```python
from build123d import *

# Parameters (mm, degrees)
EXTRUDE_F_DEPTH    = 736.6
CUT_EXTRUDE1_REACH = 740.684
SKETCH2_R          = 2.667


with BuildPart() as part:
    # Sketch1 → Extrude f (new body)
    with BuildSketch(Plane.XY):
        Polygon((3.175, 3.175), (3.175, 25.4), (0, 25.4), (0, 0), (50.8, 0), (50.8, 25.4), (47.625, 25.4), (47.625, 3.175), align=None)
    extrude(amount=EXTRUDE_F_DEPTH)

    # Sketch2 → Cut-Extrude1 (cut, up to next)
    with BuildSketch(Plane(origin=(0, 3.175, 0), x_dir=(1, 0, 0), z_dir=(0, 1, 0)), mode=Mode.PRIVATE) as cut_extrude1_sk1:
        with Locations(Location((12.7, -723.9, 0), (0, 0, 270))):
            Circle(SKETCH2_R)
    cut_extrude1_tool1 = extrude(cut_extrude1_sk1.sketch, amount=-CUT_EXTRUDE1_REACH, mode=Mode.PRIVATE) & part.part
    # Sketch2 → Cut-Extrude1 (cut, up to next)
    with BuildSketch(Plane(origin=(0, 3.175, 0), x_dir=(1, 0, 0), z_dir=(0, 1, 0)), mode=Mode.PRIVATE) as cut_extrude1_sk2:
        with Locations(Location((12.7, -660.4, 0), (0, 0, 270))):
            Circle(SKETCH2_R)
    cut_extrude1_tool2 = extrude(cut_extrude1_sk2.sketch, amount=-CUT_EXTRUDE1_REACH, mode=Mode.PRIVATE) & part.part
    # Sketch2 → Cut-Extrude1 (cut, up to next)
    with BuildSketch(Plane(origin=(0, 3.175, 0), x_dir=(1, 0, 0), z_dir=(0, 1, 0)), mode=Mode.PRIVATE) as cut_extrude1_sk3:
        with Locations(Location((38.1, -660.4, 0), (0, 0, 270))):
            Circle(SKETCH2_R)
    cut_extrude1_tool3 = extrude(cut_extrude1_sk3.sketch, amount=-CUT_EXTRUDE1_REACH, mode=Mode.PRIVATE) & part.part
    # Sketch2 → Cut-Extrude1 (cut, up to next)
    with BuildSketch(Plane(origin=(0, 3.175, 0), x_dir=(1, 0, 0), z_dir=(0, 1, 0)), mode=Mode.PRIVATE) as cut_extrude1_sk4:
        with Locations(Location((38.1, -723.9, 0), (0, 0, 270))):
            Circle(SKETCH2_R)
    cut_extrude1_tool4 = extrude(cut_extrude1_sk4.sketch, amount=-CUT_EXTRUDE1_REACH, mode=Mode.PRIVATE) & part.part
    # Sketch2 → Cut-Extrude1 (cut, up to next)
    with BuildSketch(Plane(origin=(0, 3.175, 0), x_dir=(1, 0, 0), z_dir=(0, 1, 0)), mode=Mode.PRIVATE) as cut_extrude1_sk5:
        with Locations(Location((38.1, -12.7, 0), (0, 0, 270))):
            Circle(SKETCH2_R)
    cut_extrude1_tool5 = extrude(cut_extrude1_sk5.sketch, amount=-CUT_EXTRUDE1_REACH, mode=Mode.PRIVATE) & part.part
    # Sketch2 → Cut-Extrude1 (cut, up to next)
    with BuildSketch(Plane(origin=(0, 3.175, 0), x_dir=(1, 0, 0), z_dir=(0, 1, 0)), mode=Mode.PRIVATE) as cut_extrude1_sk6:
        with Locations(Location((38.1, -76.2, 0), (0, 0, 270))):
            Circle(SKETCH2_R)
    cut_extrude1_tool6 = extrude(cut_extrude1_sk6.sketch, amount=-CUT_EXTRUDE1_REACH, mode=Mode.PRIVATE) & part.part
    # Sketch2 → Cut-Extrude1 (cut, up to next)
    with BuildSketch(Plane(origin=(0, 3.175, 0), x_dir=(1, 0, 0), z_dir=(0, 1, 0)), mode=Mode.PRIVATE) as cut_extrude1_sk7:
        with Locations(Location((12.7, -12.7, 0), (0, 0, 270))):
            Circle(SKETCH2_R)
    cut_extrude1_tool7 = extrude(cut_extrude1_sk7.sketch, amount=-CUT_EXTRUDE1_REACH, mode=Mode.PRIVATE) & part.part
    # Sketch2 → Cut-Extrude1 (cut, up to next)
    with BuildSketch(Plane(origin=(0, 3.175, 0), x_dir=(1, 0, 0), z_dir=(0, 1, 0)), mode=Mode.PRIVATE) as cut_extrude1_sk8:
        with Locations(Location((12.7, -76.2, 0), (0, 0, 270))):
            Circle(SKETCH2_R)
    cut_extrude1_tool8 = extrude(cut_extrude1_sk8.sketch, amount=-CUT_EXTRUDE1_REACH, mode=Mode.PRIVATE) & part.part
    add(cut_extrude1_tool1.solids().sort_by_distance((12.7, 3.175, 723.9))[0], mode=Mode.SUBTRACT)
    add(cut_extrude1_tool2.solids().sort_by_distance((12.7, 3.175, 660.4))[0], mode=Mode.SUBTRACT)
    add(cut_extrude1_tool3.solids().sort_by_distance((38.1, 3.175, 660.4))[0], mode=Mode.SUBTRACT)
    add(cut_extrude1_tool4.solids().sort_by_distance((38.1, 3.175, 723.9))[0], mode=Mode.SUBTRACT)
    add(cut_extrude1_tool5.solids().sort_by_distance((38.1, 3.175, 12.7))[0], mode=Mode.SUBTRACT)
    add(cut_extrude1_tool6.solids().sort_by_distance((38.1, 3.175, 76.2))[0], mode=Mode.SUBTRACT)
    add(cut_extrude1_tool7.solids().sort_by_distance((12.7, 3.175, 12.7))[0], mode=Mode.SUBTRACT)
    add(cut_extrude1_tool8.solids().sort_by_distance((12.7, 3.175, 76.2))[0], mode=Mode.SUBTRACT)


solid = part.part
```
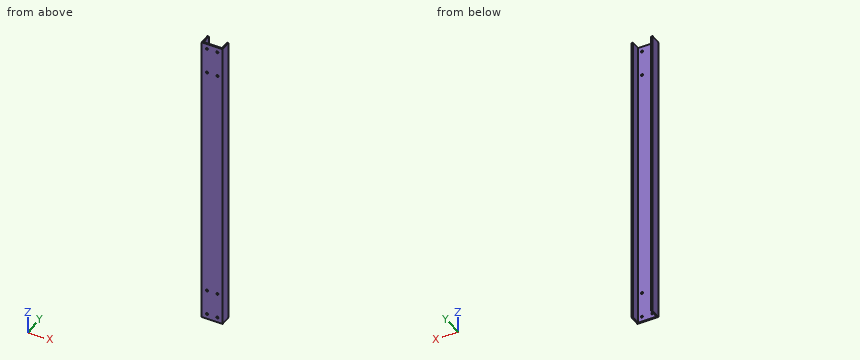
Build history of the part. All positions in model axes, mm. Give positions to 0.01 mm unless a question says otherwise; leave off trailing zeros. Loops run counter-clockwise (first coordinate to the right, second up) from the corner with the lowest first, then second, coordinate; pieces in that order, holes last. Notation, with made-up numbers: (-16.5, 50) - (19.5, 50) arc R29 ccw to (19.5, 88) - close; hole circle Ø9 at (52.25, 81.25). An arc over 180 degrees is marked (long way). Use a Markdown table: item, result.
(1) Drop flat-ended pins along their axis: pin 1 Ø7 at (x, z) = (38.1, 723.9) entering from +Y (3 decimals); pin 2 Ø7 at (x, z) = (12.7, 12.7) entering from -Y. Give the stop position or say it passes through.
Taken from the geometry:
| item | result |
|---|---|
| pin 1 | y = 3.175 |
| pin 2 | y = 0 |
(2) Band-saw the part on A-A (y = 15.25). Give the cut face in (x, z) (3 decimals), and give its area (3 significant figures).
Taken from the geometry:
| item | result |
|---|---|
| outline | (0, 0) - (3.175, 0) - (3.175, 736.6) - (0, 736.6) - close; (47.625, 0) - (50.8, 0) - (50.8, 736.6) - (47.625, 736.6) - close |
| area | 4,680 mm2 |
(3) Wall check: line 1 along X through (y, z) = (0.75, 12.7); line 2 along X through (y, z) = (7.75, 296) (3 decimals); line 3 along Y through (x, z) = (47, 688.5) (3 decimals). Give the ranges that are in metal, low to high.
Taken from the geometry:
| item | result |
|---|---|
| line 1 | 0 to 10.03, 15.37 to 35.43, 40.77 to 50.8 |
| line 2 | 0 to 3.175, 47.625 to 50.8 |
| line 3 | 0 to 3.175 |
(4) Band-saw the part on C-C (x = 29.5). Give the cut face in (y, z) (3 decimals), and give its area (3 significant figures).
Taken from the geometry:
| item | result |
|---|---|
| outline | (0, 0) - (3.175, 0) - (3.175, 736.6) - (0, 736.6) - close |
| area | 2,340 mm2 |
(5) Band-saw the part on B-B (z = 269.5). Give the cut face in (x, y) (3 decimals).
Taken from the geometry:
| item | result |
|---|---|
| outline | (0, 0) - (50.8, 0) - (50.8, 25.4) - (47.625, 25.4) - (47.625, 3.175) - (3.175, 3.175) - (3.175, 25.4) - (0, 25.4) - close |
